Input: part model. Units: mm. Frame: model coordinates. A direction names the side the tool comes from. Give positions to 0.01 mm unless a question says otherwise; leave off trailing zeros. Loops run counter-clockwise (first coordinate to the right, second up) from the corner with the lowest first, then second, coordinate; pieces in that order, holes last. Notation, with made-up numbers: (-25.5, 54.5) - (-2.5, 54.5) arc R19 ccw to (-2.5, 67.5) - close; hole circle Ø4 at (59, 69). An arc over 180 degrees is marked (long way). Answer as a JSON object with one key per item and string values. Group by question number.
(1) Access query for faces 4 (the flat face through (6, 12, 10)), 5 (the flat face through (6, 11, 0)). Directions: +Z, -Z, +X, -X, +Y, -Y. A direction counts if a zero-diameter tool reaches every point of the face in a straight line with its end or side. Return the directions, or none.
(2) Section query B-B (x = 6). Return loops of the section in (y, z).
(3) Material intervals for L1, parallel to Z at x = 6, y = -2.2; L2, parallel to X at y = -2.05, z = 67; L3, parallel to Y at x = 10.75, z = 16, sorted ascending.
(4) Section query C-C (y = 5.75). Return loops of the section in (x, z).
(5) Pin query (flat end, axial travel): P1, Ø3, axis at x = 5, y = 21.5, coming from the +Z side; P2, Ø3, axis at x = 2.5, z = 50.5, coming from the +Y side; P3, Ø1, axis at x = 1.5, y = 18.5, coming from the -Z side. Return the tip coordinate at first contact, or that it passes through.
(6) Section query A-A (z = 47). Return loops of the section in (x, y), plus the area to 3 significant figures.
(7) Section query D-D (z = 72). Return loops of the section in (x, y).
(8) Mould query, pull axis X, two halves, no side actions, for faces 1 (the cylindrical face through (6.37, -1.48, 45.34)), 2 (the flat face through (0, -2, 38)), 3 (the flat face through (6, 0, 65)). Classes: +X half, -X half, draft (parallel to the pull), parting line (faces both ways), or undercut.
```python
from build123d import *

# Parameters (mm, degrees)
F0_W     = 3
F0_H     = 122
F1_DEPTH = 12
F2_W     = 12
F2_H     = 10
F3_DEPTH = 25
F4_R     = 1.7
F5_DEPTH = 3.001


with BuildPart() as f1:
    # F0 (on Right) → F1 (new body)
    with BuildSketch(Plane.YZ):
        with Locations((-1.5, 61)):
            Rectangle(F0_W, F0_H)
    extrude(amount=F1_DEPTH)

    # F2 (on face) → F3 (join)
    with BuildSketch(Plane(origin=(0, 0, 0), x_dir=(-1, 0, 0), z_dir=(0, 1, 0))):
        with Locations((-6, 5)):
            Rectangle(F2_W, F2_H)
    extrude(amount=F3_DEPTH)

    # F4 (on face) → F5 (cut, through all)
    with BuildSketch(Plane(origin=(0, 0, 0), x_dir=(-1, 0, 0), z_dir=(0, 1, 0))):
        with Locations((-6, 107)):
            Circle(F4_R)
        with Locations((-6, 87)):
            Circle(F4_R)
        with Locations((-6, 67)):
            Circle(F4_R)
        with Locations((-6, 47)):
            Circle(F4_R)
    extrude(amount=-F5_DEPTH, mode=Mode.SUBTRACT)


solid = f1.part
```
Recorded:
{
 "1": {"face 4": "+Z, +X, -X, +Y", "face 5": "-Z, +X, -X, +Y, -Y"},
 "2": {"outline": "(-3, 0) - (25, 0) - (25, 10) - (0, 10) - (0, 45.3) - (-3, 45.3) - close; (-3, 48.7) - (0, 48.7) - (0, 65.3) - (-3, 65.3) - close; (-3, 68.7) - (0, 68.7) - (0, 85.3) - (-3, 85.3) - close; (-3, 88.7) - (0, 88.7) - (0, 105.3) - (-3, 105.3) - close; (-3, 108.7) - (0, 108.7) - (0, 122) - (-3, 122) - close"},
 "3": {"L1": "z = 0 to 45.3, 48.7 to 65.3, 68.7 to 85.3, 88.7 to 105.3, 108.7 to 122", "L2": "x = 0 to 4.3, 7.7 to 12", "L3": "y = -3 to 0"},
 "4": {"outline": "(0, 0) - (12, 0) - (12, 10) - (0, 10) - close"},
 "5": {"P1": "stops at z = 10", "P2": "stops at y = 0", "P3": "stops at z = 0"},
 "6": {"outline": "(0, -3) - (4.3, -3) - (4.3, 0) - (0, 0) - close; (7.7, -3) - (12, -3) - (12, 0) - (7.7, 0) - close", "area": "25.8 mm^2"},
 "7": {"outline": "(0, -3) - (12, -3) - (12, 0) - (0, 0) - close"},
 "8": {"face 1": "undercut", "face 2": "-X half", "face 3": "draft"}
}
